Work out the finished part from the listing and answer in its coordinate system (mm). A direction names the side the tool comes from. Round coordinates to 2 decimals unless told otherwise and drop trailing zeros. Order: outer loops, then holes, each group sorted by start corner. A loop starts at its lowest first (then second) coordinate and runs counter-clockwise, first axis right, second up. Notation, with made-up numbers: (27.5, 47.5) - (53.5, 47.5) arc R13 cw to (53.5, 66.5) - close; hole circle Ø9 at (41, 9). An arc over 180 degrees is marked (long way). Put each result on its own line as item: value.
```python
from build123d import *

# Parameters (mm, degrees)
SKETCH1_R           = 2
SKETCH1_R_2         = 2.5
BOSS_EXTRUDE1_DEPTH = 6


with BuildPart() as part:
    # Sketch1 → Boss-Extrude1 (new body)
    with BuildSketch(Plane.XY):
        Polygon((29.343145751, 0), (60, 0), (60, -20), (60, -60), (20, -60), (0, -60), (0, -29.343145751), (0, -20), (20, -20), (20, 0), align=None)
        with Locations((50, -10)):
            Circle(SKETCH1_R, mode=Mode.SUBTRACT)
        with Locations((25, -10)):
            Circle(SKETCH1_R, mode=Mode.SUBTRACT)
        with Locations((10, -50)):
            Circle(SKETCH1_R, mode=Mode.SUBTRACT)
        with Locations((10, -25)):
            Circle(SKETCH1_R, mode=Mode.SUBTRACT)
        with Locations((48, -48.833248844)):
            Circle(SKETCH1_R_2, mode=Mode.SUBTRACT)
    extrude(amount=BOSS_EXTRUDE1_DEPTH)


solid = part.part
```
1) For faces 1 (the flat face through (10, -20, 3)), 2 (the flat face through (30, -30, 6)), determine the directions among +Z, -Z, +X, -X, +Y, -Y from which every point of the face is accessible in a straight line to the end or side of a thin tool.
Findings below:
face 1: +Z, -Z, -X, +Y
face 2: +Z, +X, -X, +Y, -Y
2) A cutting plane is placed at A-A on y = -25. Write down the section's boundary in (x, z), then the cut area to 3 significant figures.
Findings below:
outline: (0, 0) - (8, 0) - (8, 6) - (0, 6) - close; (12, 0) - (60, 0) - (60, 6) - (12, 6) - close
area: 336 mm2
3) A cutting plane is placed at B-B on x = 10. Write down the section's boundary in (y, z), then the cut area to 3 significant figures.
Findings below:
outline: (-60, 0) - (-52, 0) - (-52, 6) - (-60, 6) - close; (-48, 0) - (-27, 0) - (-27, 6) - (-48, 6) - close; (-23, 0) - (-20, 0) - (-20, 6) - (-23, 6) - close
area: 192 mm2
4) A cutting plane is placed at C-C on x = 25. Write down the section's boundary in (y, z).
Findings below:
outline: (-60, 0) - (-12, 0) - (-12, 6) - (-60, 6) - close; (-8, 0) - (0, 0) - (0, 6) - (-8, 6) - close
5) For a pull along Y with two mould halves and no side action, classify faces 3 (the flat face through (40, 0, 3)), 4 (the flat face through (20, -10, 3)), 5 (the cylindrical face through (8.4, -26.2, 3)), 6 (the flat face through (30, -60, 3)) as pulls with the +Y half, pulls with the -Y half, needs draft (parallel to the pull), parting line crosses it, or undercut.
Findings below:
face 3: pulls with the +Y half
face 4: needs draft
face 5: undercut
face 6: pulls with the -Y half
6) Straight lines are drawn through the part: L1, parallel to Y at x = 10, z = 3.65; L2, parallel to Y at x = 25, z = 3.3; L3, parallel to X at y = -6.5, z = 1.2. For each, find the intervals that lie inside material, in ascending order. Write a range as from..to.
Findings below:
L1: y = -60..-52, -48..-27, -23..-20
L2: y = -60..-12, -8..0
L3: x = 20..60
7) A cutting plane is placed at D-D on y = -10. Write down the section's boundary in (x, z), then the cut area to 3 significant figures.
Findings below:
outline: (20, 0) - (23, 0) - (23, 6) - (20, 6) - close; (27, 0) - (48, 0) - (48, 6) - (27, 6) - close; (52, 0) - (60, 0) - (60, 6) - (52, 6) - close
area: 192 mm2
8) Given pin 1 Ø4 at (x, y) = (30, -21) entering from -Z; pin 2 Ø5 at (x, y) = (11, -17) entering from +Z; pin 3 Ø1.8 at (x, z) = (7.5, 4) entering from +Y, each flat-ended and moving along its own axis, determine where each tip first touches the part or whether it passes through.
Findings below:
pin 1: stops at z = 0
pin 2: passes through
pin 3: stops at y = -20
